CAD build for the part. Positions are in the model's coordinates, mm. A direction names the side the tool comes from. Give positions to 0.01 mm unless a question says otherwise; leave off trailing zeros. Loops run counter-clockwise (first coordinate to the right, second up) from the corner with the lowest first, then second, coordinate; pieces in that order, holes last.
Item 1: Saw through at A-A on y = 37. Give the cut face in (x, z).
Item 2: Drop flat-ended pins along their axis: P1, Ø10, axis at x = -10.5, y = 45.5, coming from the +Z side; P2, Ø4, axis at y = 103, z = -21, coming from the -X side; P3, Ø15, axis at y = 69.5, z = -6.5, coming from the +X side. Give the stop position or say it passes through.
Item 3: Probe probe 1 along Z at (x, y) = (-4.5, 116.5); probe 2 along Y at (x, z) = (10.5, 2) (3 decimals). List the from-to ranges inside material, lowest first.
Item 4: Saw through at D-D on x = -26. Give the cut face in (y, z) (3 decimals).
Item 5: Which spindle directions (+Z, -Z, +X, -X, +Y, -Y) get a long thin tool onto all of the face, cutting with end or side? Do faces 1 (the flat face through (17.462, 77, 0)), 2 (the flat face through (21.431, 66, 0)), 3 (the flat face through (0, 66, 21.431)). Say none if no direction does.
Item 6: Mould opens along X. For faces 4 (the flat face through (-21, 149.225, 0)), 5 (the flat face through (-21.431, 66, 0)), 6 (the flat face through (0, 3.175, 0)) say: released by +X, released by -X, zero draft, split by the parting line, or undercut.
from build123d import *

# Parameters (mm, degrees)
SKETCH1_W           = 42.8625
SKETCH1_H           = 42.8625
BOSS_EXTRUDE1_DEPTH = 133.35
SKETCH2_R           = 31.75
BOSS_EXTRUDE2_DEPTH = 15.875
SKETCH3_W           = 34.925
SKETCH3_H           = 34.925
CUT_EXTRUDE1_DEPTH  = 146.05
FILLET1_R           = 2.54


with BuildPart() as part:
    # Sketch1 → Boss-Extrude1 (new body)
    with BuildSketch(Plane(origin=(0, 0, 0), x_dir=(1, 0, 0), z_dir=(0, 1, 0))):
        Rectangle(SKETCH1_W, SKETCH1_H)
    extrude(amount=BOSS_EXTRUDE1_DEPTH)

    # Sketch2 → Boss-Extrude2 (add)
    with BuildSketch(Plane(origin=(0, 133.35, 0), x_dir=(1, 0, 0), z_dir=(0, 1, 0))):
        with Locations(Location((0, 0, 0), (0, 0, 270))):
            Circle(SKETCH2_R)
    extrude(amount=BOSS_EXTRUDE2_DEPTH)

    # Sketch3 → Cut-Extrude1 (cut)
    with BuildSketch(Plane(origin=(0, 149.225, 0), x_dir=(1, 0, 0), z_dir=(0, 1, 0))):
        Rectangle(SKETCH3_W, SKETCH3_H)
    extrude(amount=-CUT_EXTRUDE1_DEPTH, mode=Mode.SUBTRACT)

    # Fillet1
    fillet1_edges = [part.edges().sort_by_distance(p)[0] for p in [
        (17.4625, 76.2, 17.4625),
        (17.4625, 76.2, -17.4625),
        (-17.4625, 76.2, -17.4625),
        (-17.4625, 76.2, 17.4625),
        (-21.43125, 66.675, -21.43125),
        (21.43125, 66.675, -21.43125),
        (21.43125, 66.675, 21.43125),
        (-21.43125, 66.675, 21.43125),
    ]]
    fillet(fillet1_edges, radius=FILLET1_R)


solid = part.part
Results below:
1. outline: (-21.43, -18.89) arc R2.54 ccw to (-18.89, -21.43) - (18.89, -21.43) arc R2.54 ccw to (21.43, -18.89) - (21.43, 18.89) arc R2.54 ccw to (18.89, 21.43) - (-18.89, 21.43) arc R2.54 ccw to (-21.43, 18.89) - close; hole (-17.46, -14.92) arc R2.54 ccw to (-14.92, -17.46) - (14.92, -17.46) arc R2.54 ccw to (17.46, -14.92) - (17.46, 14.92) arc R2.54 ccw to (14.92, 17.46) - (-14.92, 17.46) arc R2.54 ccw to (-17.46, 14.92) - close
2. P1: stops at z = 21.43
2. P2: stops at x = -21.43
2. P3: stops at x = 21.43
3. probe 1: z = -21.43 to -17.46, 17.46 to 21.43
3. probe 2: y = 0 to 3.175
4. outline: (133.35, -18.223) - (149.225, -18.223) - (149.225, 18.223) - (133.35, 18.223) - close
5. face 1: +Y
5. face 2: +Z, -Z, +X, -Y
5. face 3: +Z, +X, -X, -Y
6. face 4: zero draft
6. face 5: released by -X
6. face 6: undercut
